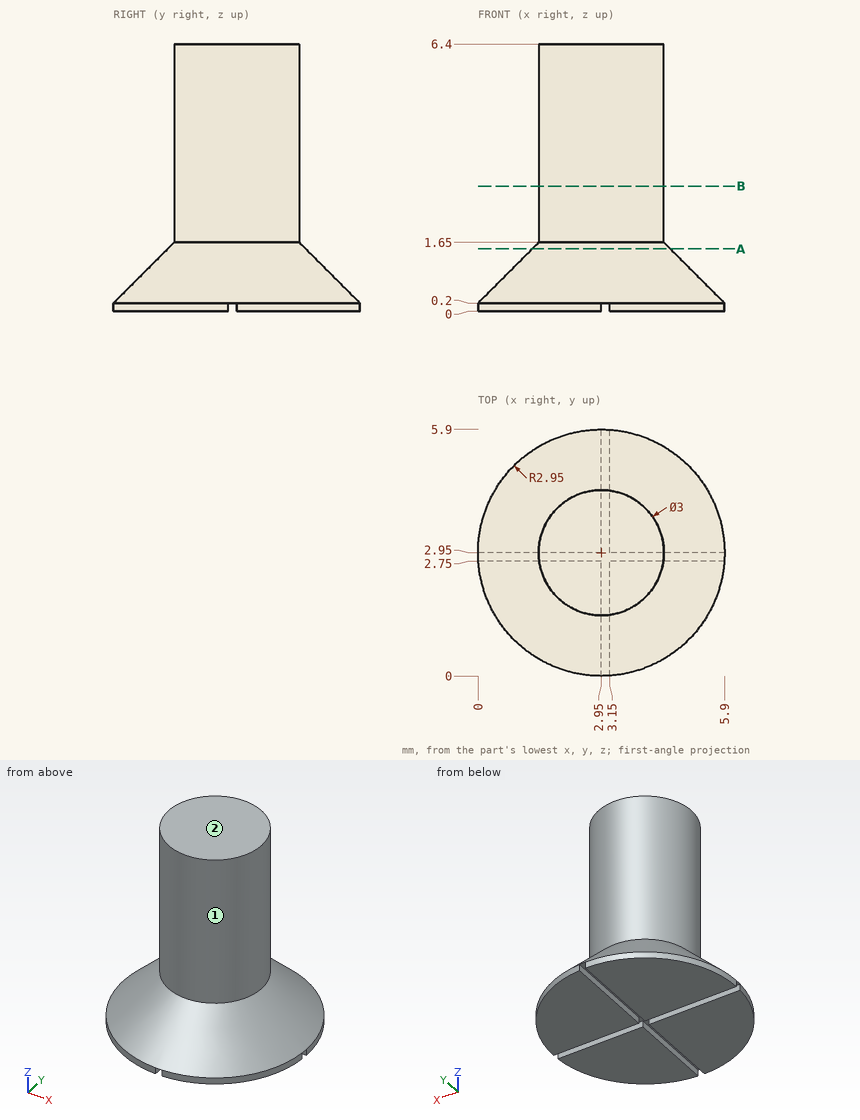
Input: dimensioned drawing with shaded views. Units: mm. Origin: part minimum x, y, z. A direction names the side the tool comes from. Coordinates: 2 decimals unless noted, no trailing zeros. Loops run counter-clockwise (first coordinate to the right, second up) from the corner with the lowest first, then second, coordinate; pieces in that order, holes last. Notation, with made-up numbers: (17, 62) - (47, 62) arc R16 cw to (47, 71) - close; hole circle Ø4 at (24.25, 20). An arc over 180 degrees is marked (long way). One line per question, with ' | ' between items. Start each with the question number.
(1) First-contact query: pin 1 (3 mm diameter, centred on x = 5, z = 1.5, fed in from +Y); pin 2 (1 mm diameter, centred on x = 3.5, z = 3.5, fed in from +Y); pin 3 (2 mm diameter, centred on y = 1.5, z = 5, fed in from -X). Flat tips, straight axial feed; report the tip coordinate or a pass-through.
(2) Ray query, L1, parallel to Y at x = 3.9, z = 1; L2, parallel to Y at x = 3.15, z = 4.25; L3, parallel to X at y = 2, z = 4.25. Return the intervals inside material, ascending. Write a range as from..to.
(3) Cut plane A-A on z = 1.5. Output: boundary loops of the cut face in (x, y), and give its area (3 significant figures).
(4) Reachability of the marked faces 1 and 2 from +Z, -Z, +X, -X, +Y, -Y: full face, straight path, thin tool, end or side. Return the list, or none.
(5) Cut plane B-B on z = 3. Output: boundary loops of the cut face in (x, y), and give its area (3 significant figures).
Here are the results:
1) pin 1: y = 5.6 | pin 2: y = 4.45 | pin 3: x = 1.52
2) L1: 1.02..4.88 | L2: 1.46..4.44 | L3: 1.79..4.11
3) outline: circle Ø3.3 at (2.95, 2.95) | area: 8.55 mm²
4) face 1: +Z | face 2: +Z, +X, -X, +Y, -Y
5) outline: circle Ø3 at (2.95, 2.95) | area: 7.07 mm²
